from build123d import *

# Parameters (mm, degrees)
SKETCH1_R           = 12.5
SKETCH1_R_2         = 1
BOSS_EXTRUDE1_DEPTH = 2
SKETCH2_R           = 4
SKETCH2_R_2         = 3
BOSS_EXTRUDE2_DEPTH = 4
SKETCH3_R           = 3
CUT_EXTRUDE1_DEPTH  = 19.668154703


with BuildPart() as part:
    # Sketch1 → Boss-Extrude1 (new body)
    with BuildSketch(Plane.XY):
        Circle(SKETCH1_R)
        with Locations((-8.5, 0)):
            Circle(SKETCH1_R_2, mode=Mode.SUBTRACT)
        with Locations((0, 8.5)):
            Circle(SKETCH1_R_2, mode=Mode.SUBTRACT)
        with Locations((8.5, 0)):
            Circle(SKETCH1_R_2, mode=Mode.SUBTRACT)
        with Locations((0, -8.5)):
            Circle(SKETCH1_R_2, mode=Mode.SUBTRACT)
    extrude(amount=BOSS_EXTRUDE1_DEPTH)

    # Sketch2 → Boss-Extrude2 (add)
    with BuildSketch(Plane.XY.offset(2)):
        Circle(SKETCH2_R)
        Circle(SKETCH2_R_2, mode=Mode.SUBTRACT)
    extrude(amount=BOSS_EXTRUDE2_DEPTH)

    # Sketch3 → Cut-Extrude1 (cut, through all)
    with BuildSketch(Plane(origin=(0, 0, 0), x_dir=(-1, 0, 0), z_dir=(0, 0, -1))):
        Circle(SKETCH3_R)
    extrude(amount=-CUT_EXTRUDE1_DEPTH, mode=Mode.SUBTRACT)


solid = part.part
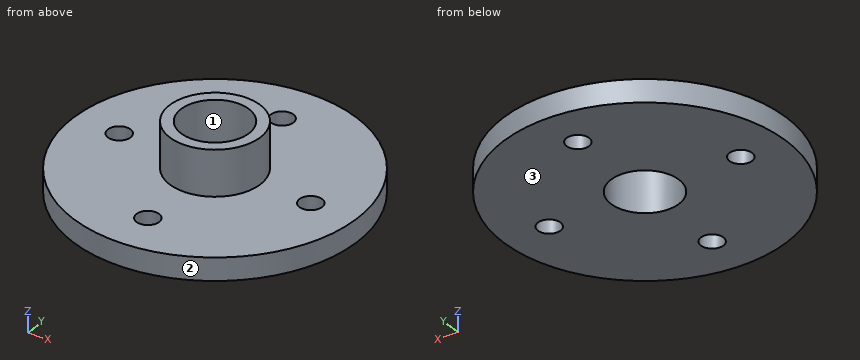
Model file for the job. Use its own axes, mm. Face numbers are marked on the shaded views. Give positions to 0.01 mm unless a question says otherwise; leave off trailing zeros. Loops run counter-clockwise (first coordinate to the right, second up) from the corner with the lowest first, then second, coordinate; pieces in that order, holes last.
Item 1: Slice it at C-C (z = 1.4). Write the cut outline in (x, y), plus the area to 3 significant figures.
Check values:
outline: circle Ø25 at (0, 0); hole circle Ø2 at (-8.5, 0); hole circle Ø6 at (0, 0); hole circle Ø2 at (0, -8.5); hole circle Ø2 at (0, 8.5); hole circle Ø2 at (8.5, 0)
area: 450 mm2
Item 2: Slice it at D-D (y = -8.5). Write the cut outline in (x, z), plus the area to 3 significant figures.
Check values:
outline: (-9.17, 0) - (-1, 0) - (-1, 2) - (-9.17, 2) - close; (1, 0) - (9.17, 0) - (9.17, 2) - (1, 2) - close
area: 32.7 mm2
Item 3: Drop flat-ended pins along their axis: P1, Ø2.5, axis at x = 8.5, y = 0, coming from the +Z side; P2, Ø2, axis at x = -1.5, z = 2.5, coming from the -Y side; P3, Ø1.2, axis at x = 0, y = 8.5, coming from the +Z side; P4, Ø1.5, axis at x = 3, z = 1, coming from the +Y side. Give the stop position or say it passes through.
Check values:
P1: stops at z = 2
P2: stops at y = -12.48
P3: passes through
P4: stops at y = 12.3
Item 4: Mould opens along X. For the marked faces 1, 2 and 3 say: +X half, -X half, draft (parallel to the pull), parting line (faces both ways), or undercut.
Check values:
face 1: undercut
face 2: parting line
face 3: draft
Item 5: Drill centre lines: line 1 along Y through (x, z) = (0, 0.95); line 2 along Z through (x, y) = (2.5, 4.25); line 3 along Y through (x, z) = (8.5, 1.05). Where is each one in solid material? Low to high.
Check values:
line 1: y = -12.5 to -9.5, -7.5 to -3, 3 to 7.5, 9.5 to 12.5
line 2: z = 0 to 2
line 3: y = -9.17 to -1, 1 to 9.17
Item 6: Slice it at A-A (y = 0). Write the cut outline in (x, z).
Check values:
outline: (-12.5, 0) - (-9.5, 0) - (-9.5, 2) - (-12.5, 2) - close; (-7.5, 0) - (-3, 0) - (-3, 6) - (-4, 6) - (-4, 2) - (-7.5, 2) - close; (3, 0) - (7.5, 0) - (7.5, 2) - (4, 2) - (4, 6) - (3, 6) - close; (9.5, 0) - (12.5, 0) - (12.5, 2) - (9.5, 2) - close
